Geometry check sheet. Reference: drawing and pictorial views, mm from the part's lowest x, y, z. Round coordinates to 2 decimals unless told otherwise and drop trailing zeros. Write each loop counter-clockwise with the first axis right and the second up, starting at its lowest first coordinate (ties: lowest second). Pieces come first, ordered by that corner, then holes. Notation, with made-up numbers: M -25,18 L 29,18 A25 ccw 29,40 Z; hole C -13.75,16 d10. An arc over 180 degrees is marked long. Answer in a Markdown table with one row per item.
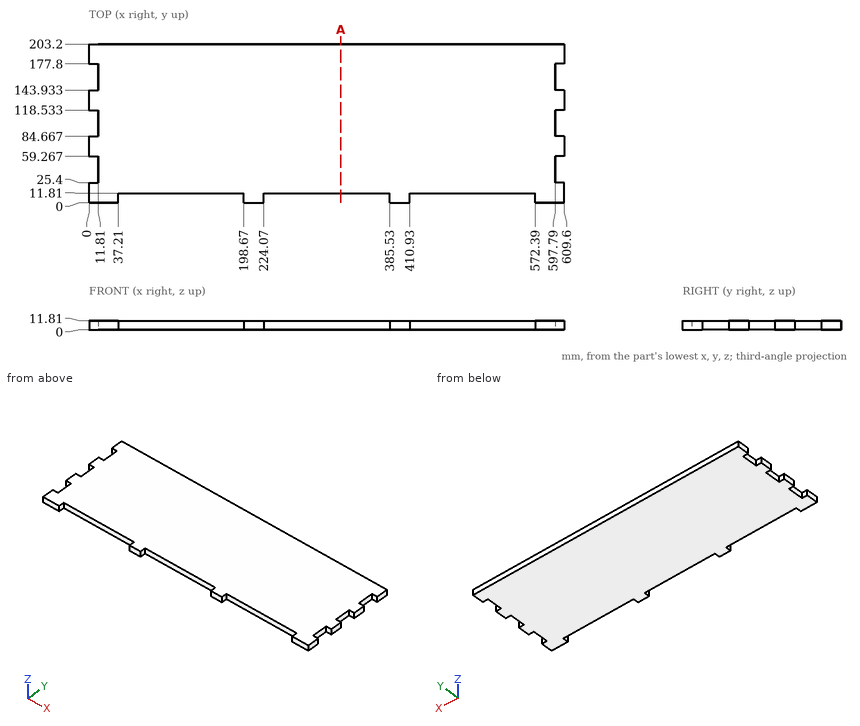
1. Go/stop test with flat-tipped pins: pin 1 (2 mm diameter, centred on x = 246.5, y = 162, fed in from -Z); pin 2 (3.5 mm diameter, centred on x = 308, z = 6, fed in from -Y); pin 3 (6 mm diameter, centred on y = 32, z = 2, fed in from -X). Record where each tip stops, or that it passes through.
Found:
| item | result |
|---|---|
| pin 1 | stops at z = 0 |
| pin 2 | stops at y = 11.81 |
| pin 3 | stops at x = 11.81 |
2. Section check A-A, the plane x = 323. Record the cut outline in (y, z), and give its area (3 significant figures).
Found:
| item | result |
|---|---|
| outline | M 11.81,0 L 203.2,0 L 203.2,11.81 L 11.81,11.81 Z |
| area | 2,260 mm2 |
3. Scan lines: L1, parallel to Y at x = 422, z = 10; L2, parallel to X at y = 28.5, z = 1.75. Record each from-to range of solid material in increasing order.
Found:
| item | result |
|---|---|
| L1 | y = 11.81 to 203.2 |
| L2 | x = 11.81 to 597.79 |
